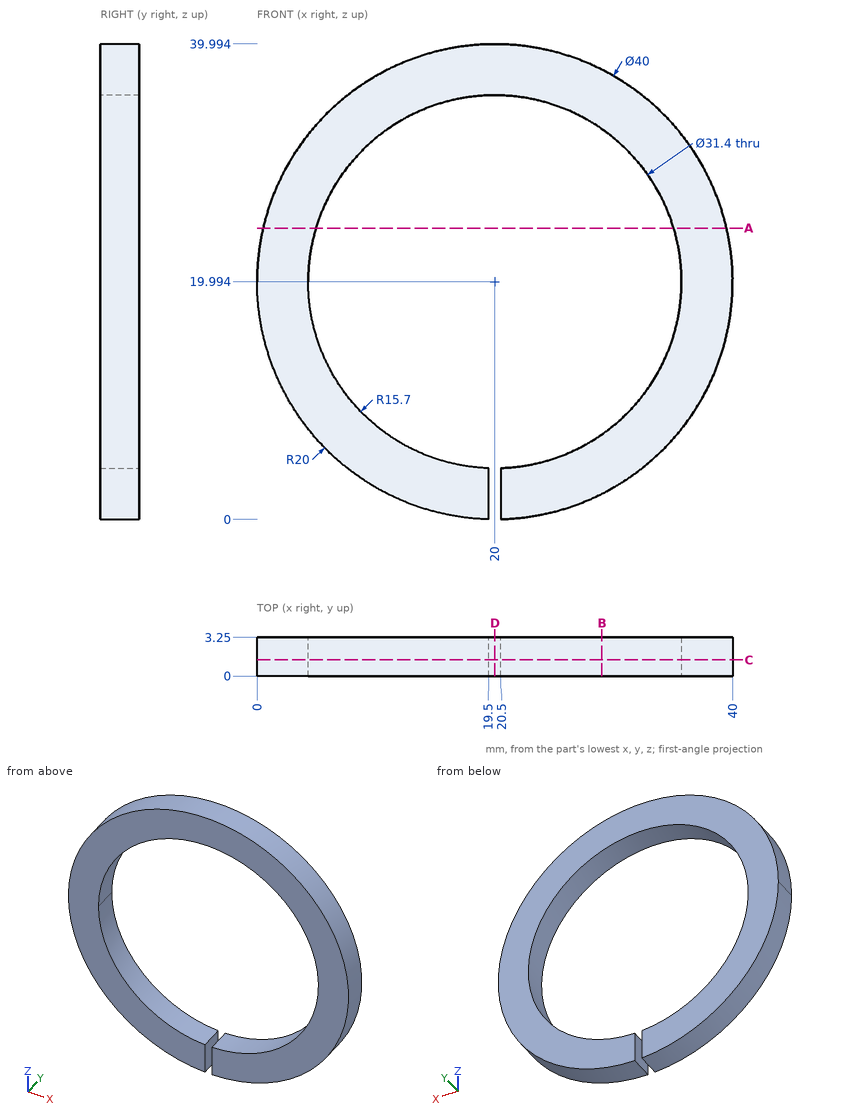
Drawing for the job (mm, zero at the part's lowest x, y, z). Round coordinates to 2 decimals unless told otherwise and drop trailing zeros. Write each loop counter-clockwise with the first axis right and the second up, starting at its lowest first coordinate (ties: lowest second). Pieces come first, ordered by that corner, then holes. Notation, with made-up numbers: (64.5, 52.5) - (117.5, 52.5) arc R22 cw to (117.5, 72.5) - close; hole circle Ø8 at (56.25, 49.25). An arc over 180 degrees is marked (long way). Use CSV: the item, a comma, the result in double quotes.
(1) Wall check: line 1 (X direction, y = 1.6, z = 19.5); line 2 (Z direction, x = 20, y = 0.9); line 3 (X direction, y = 0.85, z = 9). Give the ranges that are in metal, low to high.
Response:
line 1,"0.01 to 4.31, 35.69 to 39.99"
line 2,"35.69 to 39.99"
line 3,"3.29 to 8.79, 31.21 to 36.71"
(2) Band-saw the part on A-A (z = 24.5). Write the cut outline in (x, y), plus the area to 3 significant figures.
Response:
outline,"(0.51, 0) - (4.96, 0) - (4.96, 3.25) - (0.51, 3.25) - close; (35.04, 0) - (39.49, 0) - (39.49, 3.25) - (35.04, 3.25) - close"
area,"28.9 mm²"
(3) Band-saw the part on B-B (x = 29). Write the cut outline in (y, z).
Response:
outline,"(0, 2.13) - (3.25, 2.13) - (3.25, 7.13) - (0, 7.13) - close; (0, 32.86) - (3.25, 32.86) - (3.25, 37.85) - (0, 37.85) - close"
(4) Band-saw the part on C-C (y = 1.35). Write the cut outline in (x, z).
Response:
outline,"(19.5, 0) - (19.5, 4.3) arc R15.7 cw (long way) to (20.5, 4.3) - (20.5, 0) arc R20 ccw (long way) to start"
(5) Band-saw the part on D-D (x = 20). Write the cut outline in (y, z), plus the area to 3 significant figures.
Response:
outline,"(0, 35.69) - (3.25, 35.69) - (3.25, 39.99) - (0, 39.99) - close"
area,"14.0 mm²"
